from build123d import *

# Parameters (mm, degrees)
SKETCH2_W           = 100
SKETCH2_H           = 50
SKETCH2_R           = 5
BOSS_EXTRUDE1_DEPTH = 2
SKETCH5_W           = 2
SKETCH5_H           = 7
CUT_EXTRUDE3_DEPTH  = 2
CUT_EXTRUDE6_DEPTH  = 2
SKETCH11_W          = 5
SKETCH11_H          = 2
CUT_EXTRUDE7_DEPTH  = 2
SKETCH12_W          = 6.5
SKETCH12_H          = 50
SKETCH12_W_2        = 2.8
CUT_EXTRUDE8_DEPTH  = 6
SKETCH13_W          = 12
SKETCH13_H          = 50
SKETCH13_W_2        = 2
SKETCH13_H_2        = 7
SKETCH13_W_3        = 5
SKETCH13_H_3        = 2
CUT_EXTRUDE10_DEPTH = 6


with BuildPart() as part:
    # Sketch2 → Boss-Extrude1 (new body)
    with BuildSketch(Plane(origin=(0, 0, 0), x_dir=(1, 0, 0), z_dir=(0, 1, 0))):
        Rectangle(SKETCH2_W, SKETCH2_H)
        with Locations(Location((0, 0, 0), (0, 0, 270))):
            Circle(SKETCH2_R, mode=Mode.SUBTRACT)
    extrude(amount=BOSS_EXTRUDE1_DEPTH)

    # Sketch5 → Cut-Extrude3 (cut)
    with BuildSketch(Plane(origin=(0, 0, 0), x_dir=(-1, 0, 0), z_dir=(0, -1, 0))):
        with Locations((-24.2, -15.5)):
            Rectangle(SKETCH5_W, SKETCH5_H)
        with Locations((-24.2, 0)):
            Rectangle(SKETCH5_W, SKETCH5_H)
        with Locations((-24.2, 15.5)):
            Rectangle(SKETCH5_W, SKETCH5_H)
        with Locations((10.5, 15.5)):
            Rectangle(SKETCH5_W, SKETCH5_H)
        with Locations((10.5, 0)):
            Rectangle(SKETCH5_W, SKETCH5_H)
        with Locations((10.5, -15.5)):
            Rectangle(SKETCH5_W, SKETCH5_H)
    extrude(amount=-CUT_EXTRUDE3_DEPTH, mode=Mode.SUBTRACT)

    # Sketch10 → Cut-Extrude6 (cut)
    with BuildSketch(Plane(origin=(0, 2, 0), x_dir=(1, 0, 0), z_dir=(0, 1, 0))):
        with BuildLine():
            ThreePointArc((-5.171573663, 23.436186248), (5.745726742, 23.302073389), (15.473926709, 18.345506049))
            Line((15.473926709, 18.345506049), (7.092216408, 8.408356939))
            ThreePointArc((7.092216408, 8.408356939), (1.811815129, 10.849761561), (-3.975341771, 10.256542195))
            Line((-3.975341771, 10.256542195), (-5.171573663, 23.436186248))
        make_face()
    extrude(amount=-CUT_EXTRUDE6_DEPTH, mode=Mode.SUBTRACT)

    # Sketch11 → Cut-Extrude7 (cut)
    with BuildSketch(Plane(origin=(0, 2, 0), x_dir=(1, 0, 0), z_dir=(0, 1, 0))):
        with Locations((32.7, 22)):
            Rectangle(SKETCH11_W, SKETCH11_H)
        with Locations((-19, 22)):
            Rectangle(SKETCH11_W, SKETCH11_H)
        with Locations((-19, -22)):
            Rectangle(SKETCH11_W, SKETCH11_H)
        with Locations((32.7, -22)):
            Rectangle(SKETCH11_W, SKETCH11_H)
    extrude(amount=-CUT_EXTRUDE7_DEPTH, mode=Mode.SUBTRACT)

    # Sketch12 → Cut-Extrude8 (cut)
    with BuildSketch(Plane(origin=(0, 2, 0), x_dir=(1, 0, 0), z_dir=(0, 1, 0))):
        with Locations((-46.75, 0)):
            Rectangle(SKETCH12_W, SKETCH12_H)
        with Locations((48.6, 0)):
            Rectangle(SKETCH12_W_2, SKETCH12_H)
    extrude(amount=-CUT_EXTRUDE8_DEPTH, mode=Mode.SUBTRACT)

    # Sketch13 → Cut-Extrude10 (cut)
    with BuildSketch(Plane(origin=(0, 2, 0), x_dir=(1, 0, 0), z_dir=(0, 1, 0))):
        with Locations((41.2, 0)):
            Rectangle(SKETCH13_W, SKETCH13_H)
        with Locations((30.2, 15.5)):
            Rectangle(SKETCH13_W_2, SKETCH13_H_2)
        with Locations((30.2, -15.5)):
            Rectangle(SKETCH13_W_2, SKETCH13_H_2)
        with Locations((30.2, 0)):
            Rectangle(SKETCH13_W_2, SKETCH13_H_2)
        Polygon((-28.2, 12), (-28.2, 19), (-30.2, 19), (-30.2, 25), (-43.5, 25), (-43.5, -25), (-30.2, -25), (-30.2, -19), (-28.2, -19), (-28.2, -12), (-30.2, -12), (-30.2, -3.5), (-28.2, -3.5), (-28.2, 3.5), (-30.2, 3.5), (-30.2, 12), align=None)
        with Locations((21.7, -24)):
            Rectangle(SKETCH13_W_3, SKETCH13_H_3)
        with Locations((21.7, 24)):
            Rectangle(SKETCH13_W_3, SKETCH13_H_3)
        with Locations((-20.7, 24)):
            Rectangle(SKETCH13_W_3, SKETCH13_H_3)
        with Locations((-20.7, -24)):
            Rectangle(SKETCH13_W_3, SKETCH13_H_3)
    extrude(amount=-CUT_EXTRUDE10_DEPTH, mode=Mode.SUBTRACT)


solid = part.part
The listing builds one solid part. Answer for the finished solid, in the listing's coordinates (mm). A direction names the side the tool comes from. Round coordinates to 2 decimals unless told otherwise and drop trailing zeros. Order: outer loops, then holes, each group sorted by start corner. A loop starts at its lowest first (then second) coordinate and runs counter-clockwise, first axis right, second up. Notation, with made-up numbers: M 24.25,-14.75 L 32.25,-14.75 A23 cw 32.25,-3.75 Z; hole C -37.75,60.5 d8. An arc over 180 degrees is marked long. Answer in a Markdown table with one row per item. Add a question column.
1) Flat-ended cylindrical pins translate along their axes: pin 1 Ø8 at (x, z) = (0, 0) entering from +Y; pin 2 Ø1 at (y, z) = (1.5, 14) entering from -X; pin 3 Ø12 at (x, z) = (21.5, 8.5) entering from -Y. Find the tip coordinate at first contact, or state that the pin passes through.
2) Determine the mould class of faces 1 (the face through (-10, 1, 3.5)), 2 (the face through (30.2, 1, 22)), 3 (the face through (30, 1, -25)), 4 (the face through (-11.5, 1, 16)) for opening direction X: pulls with the +X half, pulls with the -X half, needs draft (parallel to the pull), parting line crosses it, or undercut.
3) Consider line 1 along X through (y, z) = (0.9, 0); line 2 along X through (y, z) = (0.95, 14); line 3 along Z through (x, y) = (13, 1.8). Determine where each line is inside the solid, lowest interval first. Write a range as from..to.
4) The part is cut by section D-D on y = 0.5. Count the separate pieces of the cut face and the enclosed holes in it, plus the area to 3 significant figures.
5) The part is cut by section A-A on x = 0. Determine the outline of the cut face in (y, z).
6) The part is cut by section C-C on z = 13. Determine the outline of the cut face in (x, y), plus the area to 3 significant figures.
7) The part is cut by section B-B on z = 0. Determine the outline of the cut face in (x, y), plus the area to 3 significant figures.
8) Which of the six approach directions +Z, -Z, +X, -X, +Y, -Y give full straight-line access (tool end or side, diameter ignored) to faces 5 (the face through (-23.2, 1, 24)), 6 (the face through (-27, 1, 25)), 7 (the face through (-10, 1, -3.5)), 8 (the face through (-29, 1, -19)), 9 (the face through (19.2, 1, -24))?
Findings below:
| question | item | result |
|---|---|---|
| 1 | pin 1 | passes through |
| 1 | pin 2 | stops at x = -28.2 |
| 1 | pin 3 | stops at y = 0 |
| 2 | face 1 | undercut |
| 2 | face 2 | pulls with the +X half |
| 2 | face 3 | needs draft |
| 2 | face 4 | undercut |
| 3 | line 1 | x = -28.2..-11.5, -9.5..-5, 5..23.2, 25.2..29.2, 31.2..35.2 |
| 3 | line 2 | x = -28.2..-11.5, -9.5..23.2, 25.2..29.2, 31.2..35.2 |
| 3 | line 3 | z = -25..-20.17, -15.41..25 |
| 4 | separate pieces | 1 |
| 4 | enclosed holes | 11 |
| 4 | area | 2,720 mm² |
| 5 | outline | M 0,-25 L 2,-25 L 2,-24 L 0,-24 Z; M 0,-11 L 2,-11 L 2,-5 L 0,-5 Z; M 0,5 L 2,5 L 2,25 L 0,25 Z |
| 6 | outline | M -28.2,0 L -11.5,0 L -11.5,2 L -28.2,2 Z; M -9.5,0 L 23.2,0 L 23.2,2 L -9.5,2 Z; M 25.2,0 L 29.2,0 L 29.2,2 L 25.2,2 Z; M 31.2,0 L 35.2,0 L 35.2,2 L 31.2,2 Z |
| 6 | area | 115 mm² |
| 7 | outline | M -28.2,0 L -11.5,0 L -11.5,2 L -28.2,2 Z; M -9.5,0 L -5,0 L -5,2 L -9.5,2 Z; M 5,0 L 23.2,0 L 23.2,2 L 5,2 Z; M 25.2,0 L 29.2,0 L 29.2,2 L 25.2,2 Z; M 31.2,0 L 35.2,0 L 35.2,2 L 31.2,2 Z |
| 7 | area | 94.8 mm² |
| 8 | face 5 | +Z, +Y, -Y |
| 8 | face 6 | +Z, +X, -X, +Y, -Y |
| 8 | face 7 | +Y, -Y |
| 8 | face 8 | -X, +Y, -Y |
| 8 | face 9 | -Z, +Y, -Y |
